The drawing under review shows one solid part. Ordinate dimensions are in mm from its lowest x, y, z. A direction names the side the tool comes from. Round coordinates to 2 decimals unless told otherwise and drop trailing zeros. Order: outer loops, then holes, each group sorted by start corner. A loop starts at its lowest first (then second) coordinate and runs counter-clockwise, first axis right, second up. Notation, with made-up numbers: M 20.25,25.5 L 45.25,25.5 A17 cw 45.25,55.5 Z; hole C 56,71.25 d6. An arc over 180 degrees is marked long. Answer as a JSON object with one key per item and string values. Group by question number.
1. Mouldability with a two-part tool opening along Y and no side actions: class the marked faces 1, 2 and 3 as released by +Y, released by -Y, zero draft, split by the parting line, or undercut.
2. Add section C-C on y = 7. State the section outline as (x, z) points, and give its area (3 significant figures).
3. Clearance check with flat-ended pins moving along their axes: P1, Ø8, axis at x = 12, z = 2.5, coming from the -Y side; P2, Ø2.5, axis at y = 7, z = 6.5, coming from the +X side. State where each tip first meets the part, or that it passes through.
4. Add section A-A on x = 25. State the section outline as (y, z) points, and give its area (3 significant figures).
5. Add section D-D on z = 7.5. State the section outline as (x, y) points.
6. To check wall thickness, follow probe 1 along Y at (x, z) = (31, 7.5); probe 2 along Y at (x, z) = (30, 9); probe 3 along Z at (x, y) = (8.5, 62.75). State the ranges of each line that lie inside material, in increasing order. Write a range as [from, to].
7. Add section B-B on x = 8.5. State the section outline as (y, z) points, and give its area (4 significant figures).
8. Machinability: for the marked faces 4 and 5, which of the approach directions +Z, -Z, +X, -X, +Y, -Y give a long, thin tool a straight path to every point of the face, cutting with its end or side? Answer none if there is none.
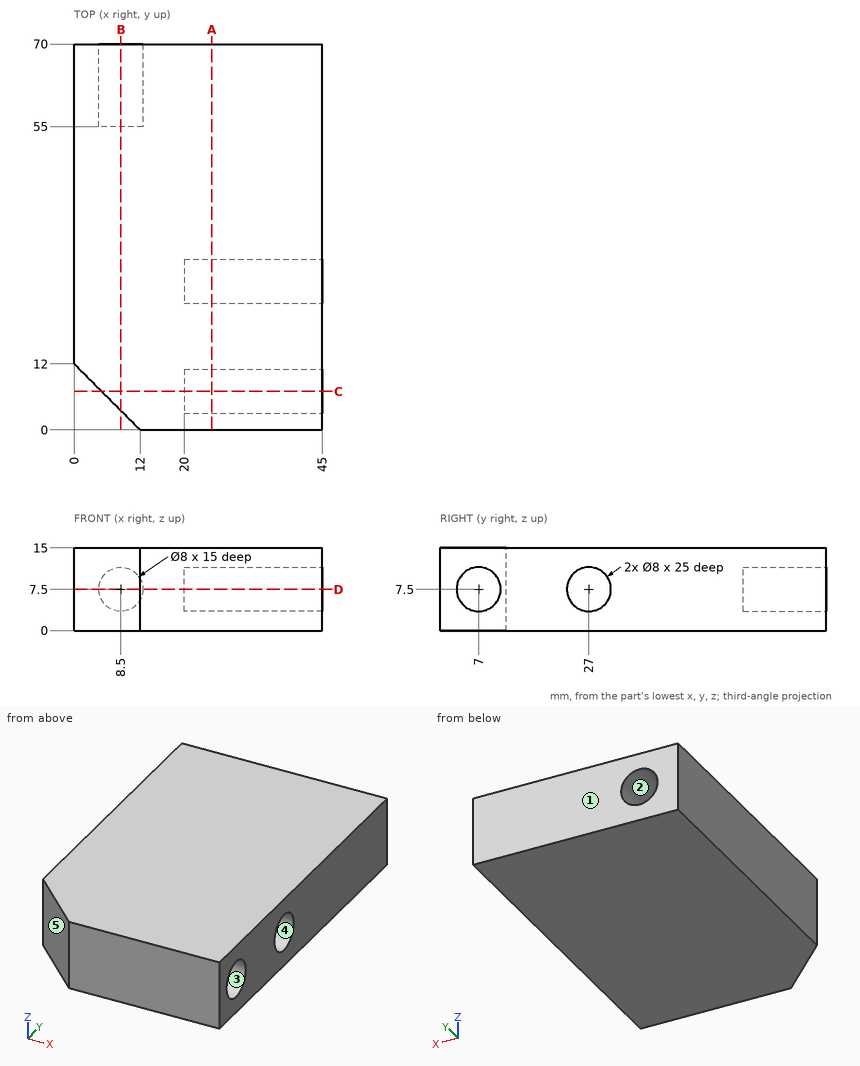
Recorded:
{
 "1": {"face 1": "released by +Y", "face 2": "zero draft", "face 3": "undercut"},
 "2": {"outline": "M 5,0 L 45,0 L 45,3.5 L 20,3.5 L 20,11.5 L 45,11.5 L 45,15 L 5,15 Z", "area": "400 mm²"},
 "3": {"P1": "stops at y = 0", "P2": "stops at x = 20"},
 "4": {"outline": "M 0,0 L 70,0 L 70,15 L 0,15 Z; hole C 7,7.5 d8; hole C 27,7.5 d8", "area": "949 mm²"},
 "5": {"outline": "M 0,12 L 12,0 L 45,0 L 45,3 L 20,3 L 20,11 L 45,11 L 45,23 L 20,23 L 20,31 L 45,31 L 45,70 L 12.5,70 L 12.5,55 L 4.5,55 L 4.5,70 L 0,70 Z"},
 "6": {"probe 1": "y = [0, 3], [11, 23], [31, 70]", "probe 2": "y = [0, 3.29], [10.71, 23.29], [30.71, 70]", "probe 3": "z = [0, 3.5], [11.5, 15]"},
 "7": {"outline": "M 3.5,0 L 70,0 L 70,3.5 L 55,3.5 L 55,11.5 L 70,11.5 L 70,15 L 3.5,15 Z", "area": "877.5 mm²"},
 "8": {"face 4": "+X", "face 5": "+Z, -Z, -X, -Y"}
}
